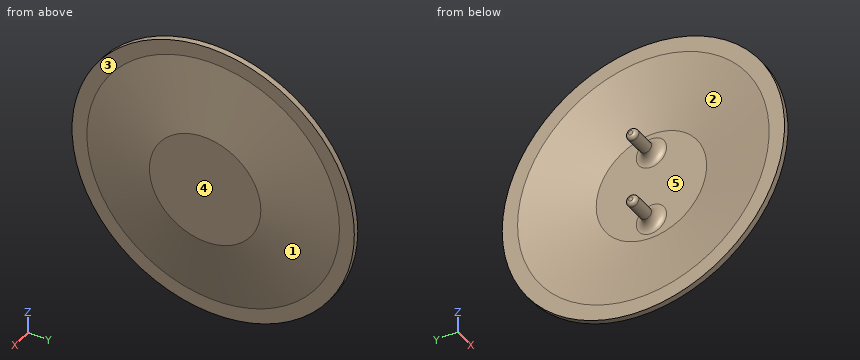
```python
from build123d import *

# Parameters (mm, degrees)
AUFSATZ_LINEAR_START            = 3.5
SKIZZE2_R                       = 1.575
AUFSATZ_LINEAR_AUSTRAGEN1_DEPTH = 9
VERRUNDUNG1_R                   = 1
VERRUNDUNG2_R                   = 2.5


with BuildPart() as part:
    # Skizze1 → Rotation1 (revolve)
    with BuildSketch(Plane.XY):
        Polygon((0, 33.862994677), (0, 38), (1.5, 38), (1.5, 34), (5, 15), (5, 0), (3.5, 0), (3.5, 14.862994677), align=None)
    revolve(axis=Axis((0, 0, 0), (1, 0, 0)))

    # Skizze2 → Aufsatz-Linear austragen1 (add)
    with BuildSketch(Plane(origin=(0, 0, 0), x_dir=(0, 0, -1), z_dir=(1, 0, 0)).offset(AUFSATZ_LINEAR_START)):
        with Locations((9.525, 0)):
            Circle(SKIZZE2_R)
        with Locations((-9.525, 0)):
            Circle(SKIZZE2_R)
    extrude(amount=-AUFSATZ_LINEAR_AUSTRAGEN1_DEPTH)

    # Verrundung1
    verrundung1_edges = [part.edges().sort_by_distance(p)[0] for p in [
        (-5.5, 0, -7.95),
        (-5.5, 0, 11.1),
    ]]
    fillet(verrundung1_edges, radius=VERRUNDUNG1_R)

    # Verrundung2
    verrundung2_edges = [part.edges().sort_by_distance(p)[0] for p in [
        (3.5, 0, -7.95),
        (3.5, 0, 11.1),
    ]]
    fillet(verrundung2_edges, radius=VERRUNDUNG2_R)


solid = part.part
```
Design review of the part built by this model. Coordinates are the model's own, in mm. Face numbers are marked on the shaded views. A direction names the side the tool comes from. Give positions to 0.01 mm unless a question says otherwise; leave off trailing zeros. Write each loop counter-clockwise with the first axis right and the second up, starting at its lowest first coordinate (ties: lowest second). Pieces come first, ordered by that corner, then holes. Notation, with made-up numbers: (-8, 43.5) - (39, 43.5) arc R12 cw to (39, 64.5) - close; hole circle Ø7 at (41.25, 14.25). An arc over 180 degrees is marked (long way). Return JSON: item names as keys, results as strings. Group by question number.
(1) To check wall thickness, follow probe 1 along X at (y, z) = (-11, -2); probe 2 along X at (y, z) = (-27.5, -24.5). State the ranges of each line that lie inside material, in increasing order.
(2) Machinability: for the marked faces 4 and 5, which of the approach directions +Z, -Z, +X, -X, +Y, -Y give a long, thin tool a straight path to every point of the face, cutting with its end or side? Answer none if there is none.
(3) We need section A-A, the plane z = 0. Give the boundary of the cut face in (x, y).
(4) Insertion check: pin 1 (5 mm diameter, centred on x = -0.5, y = 3.5, fed in from -Z); pin 2 (3 mm diameter, centred on x = 1, y = -3.5, fed in from -Z); pin 3 (4 mm diameter, centred on y = -7, z = 6.5, fed in from -X). Each pin has a flat end and moves straight along its axis. Give the tip position at first contact, or say it passes through.
(5) Mouldability with a two-part tool opening along Y and no side actions: class the marked faces 1, 2 and 3 as +Y half, -Y half, draft (parallel to the pull), parting line (faces both ways), or undercut.
Reported:
{
 "1": {"probe 1": "x = 3.5 to 5", "probe 2": "x = 0 to 1.5"},
 "2": {"face 4": "+Z, -Z, +X, +Y, -Y", "face 5": "-X"},
 "3": {"outline": "(0, -38) - (1.5, -38) - (1.5, -34) - (5, -15) - (5, 15) - (1.5, 34) - (1.5, 38) - (0, 38) - (0, 33.86) - (3.5, 14.86) - (3.5, -14.86) - (0, -33.86) - close"},
 "4": {"pin 1": "stops at z = -37.99", "pin 2": "stops at z = -37.95", "pin 3": "stops at x = 3.5"},
 "5": {"face 1": "parting line", "face 2": "undercut", "face 3": "draft"}
}
